```python
from build123d import *

# Parameters (mm, degrees)
EXTRUDE_DEPTH = 10


with BuildPart() as part:
    # Sketch → Extrude (new body)
    with BuildSketch(Plane.XY):
        with BuildLine():
            Line((-3.696471, -10.672124), (-0.696471, -10.672124))
            Line((-0.696471, -10.672124), (-0.696471, -5.672124))
            Line((-0.696471, -5.672124), (0.303529, -5.672124))
            ThreePointArc((6.795663, 5.782347), (2.039411, 0.91105), (0.303529, -5.672124))
            ThreePointArc((6.795663, 5.782347), (7.484095, 8.525714), (4.740728, 9.214146))
            ThreePointArc((4.740728, 9.214146), (-1.440512, 2.883392), (-3.696471, -5.672124))
            Line((-3.696471, -5.672124), (-3.696471, -10.672124))
        make_face()
    extrude(amount=EXTRUDE_DEPTH)


solid = part.part
```
Geometry: final body of the model. Coordinates: model frame, mm. A direction names the side the tool comes from. Coordinates: 2 decimals unless noted, no trailing zeros. Order: outer loops, then holes, each group sorted by start corner. A loop starts at its lowest first (then second) coordinate and runs counter-clockwise, first axis right, second up. Notation, with made-up numbers: (45.25, 68) - (57.25, 68) arc R19 cw to (57.25, 98) - close; hole circle Ø2 at (35, -3.75). An arc over 180 degrees is marked (long way). Write each question's results on one line, items separated by ' | '.
1) Set-up query: faces 1 (the flat face through (0, -5.672, 5)), 2 (the flat face through (-3.696, -8, 5)). Return all of +Z, -Z, +X, -X, +Y, -Y with unobstructed straight access to the full face (end or side cutting, diameter ignored); none if empty.
Results list:
face 1: +Z, -Z, +X, -Y | face 2: +Z, -Z, -X, +Y, -Y
2) Section C-C, the plane x = 1.5. Return loops of the section in (y, z).
Results list:
outline: (-0.15, 0) - (6.71, 0) - (6.71, 10) - (-0.15, 10) - close
3) Pin query (flat end, axial travel): pin 1 (5.5 mm diameter, centred on y = -7.5, z = 7.5, fed in from +X); pin 2 (6 mm diameter, centred on x = 6, z = 5.5, fed in from -Y); pin 3 (1.1 mm diameter, centred on x = 0, z = 6.5, fed in from -Y). Return the tip coordinate at first contact, or that it passes through.
Results list:
pin 1: x = 0.34 | pin 2: y = 2.37 | pin 3: y = -5.67
4) Section B-B, the plane y = -7.75. Return loops of the section in (x, z).
Results list:
outline: (-3.7, 0) - (-0.7, 0) - (-0.7, 10) - (-3.7, 10) - close
5) Line query: line 1 (X direction, y = -7.75, z = 2.25); line 2 (X direction, y = -0.25, z = 6); line 3 (Y direction, x = 3, z = 4.75). Output: solid intervals per line, ascending. Write a range as from..to.
Results list:
line 1: -3.7..-0.7 | line 2: -2.83..1.45 | line 3: 2.37..8.02
6) Section A-A, the plane z = 7.5. Return loops of the section in (x, y), plus the area to 3 significant figures.
Results list:
outline: (-3.7, -10.67) - (-0.7, -10.67) - (-0.7, -5.67) - (0.3, -5.67) arc R13.35 cw to (6.8, 5.78) arc R2 ccw to (4.74, 9.21) arc R17.35 ccw to (-3.7, -5.67) - close | area: 84.6 mm^2
